Autodesk Inventor part; units mm, degrees
ref_plane "Work Plane1" through (-16.584, 2, -16.584) normal (0, 1, 0) x (0.3814, 0, 0.9244)
ref_plane "YZ Plane" through (0, 0, 0) normal (1, 0, 0) x (0, 1, 0)
ref_plane "XZ Plane" through (0, 0, 0) normal (0, 1, 0) x (-1, 0, 0)
ref_plane "Work Plane1" through (-16.584, 2, -16.584) normal (0, 1, 0) x (0.3814, 0, 0.9244)
sketch "Sketch1" plane through (0, 0, 0) normal (0, 1, 0) x (-1, 0, 0)
  circle A0 centre (0, 0) radius 22.5
  circle A1 centre (0, 0) radius 19.5
  circle A2 centre (0, 0) radius 12.7
  circle A3 centre (0, 0) radius 6
  circle A4 centre (8.8049, 3.6331) radius 1.63
  circle A5 centre (7.5488, -5.8087) radius 1.63
  circle A6 centre (-1.2561, -9.4418) radius 1.63
  circle A7 centre (-8.8049, -3.6331) radius 1.63
  circle A8 centre (-7.5488, 5.8087) radius 1.63
  circle A9 centre (1.2561, 9.4418) radius 1.63
  circle A10 centre (0, 0) radius 12.85
  dimension "d0" = 45
  dimension "d1" = 3
  dimension "d4" = 0.15
extrude "Extrusion1" add sketch "Sketch1" along normal blind 2 contours A1
sketch "Sketch4" plane through (0, 2, 0) normal (0, 1, 0) x (1, 0, 0)
  circle A0 centre (0, 0) radius 22.5
  circle A1 centre (0, 0) radius 19.5
  circle A2 centre (0, 0) radius 18.5
  dimension "d13" = 45
  dimension "d14" = 3
  dimension "d15" = 1
extrude "Extrusion4" add sketch "Sketch4" along normal blind 51 contours A1
fillet "Fillet2" radius 1 1 edges at (12.85, 0, 0)
fillet "Fillet3" radius 2 1 edges at (-18.5, 2, 0)
properties part number "tulejka"
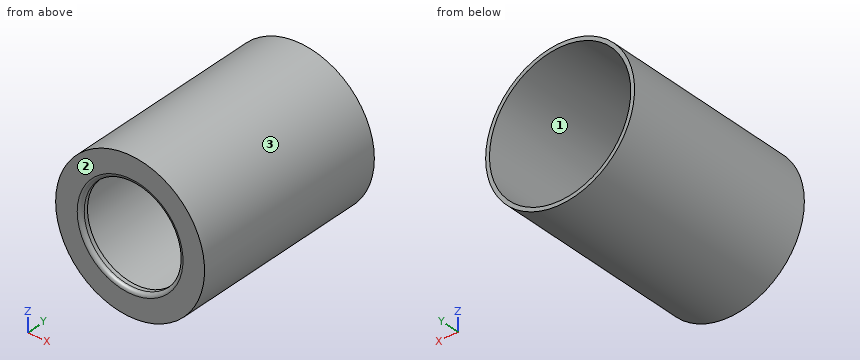
CAD build for the part. Positions are in the model's coordinates, mm. Face numbers are marked on the shaded views. Give positions to 0.01 mm unless a question says otherwise; leave off trailing zeros. Write each loop counter-clockwise with the first axis right and the second up, starting at its lowest first coordinate (ties: lowest second). Pieces come first, ordered by that corner, then holes. Notation, with made-up numbers: (81, -40) - (88, -40) arc R20 cw to (88, -19) - close; hole circle Ø6 at (35.5, -19). An arc over 180 degrees is marked (long way). Put each result on its own line as item: value.
(1) Wall check: L1, parallel to Z at x = 0, y = 1.5; L2, parallel to X at y = 33, z = 0. Give the ranges that are in metal, low to high.
Working result:
L1: -19.5 to -12.85, 12.85 to 19.5
L2: -19.5 to -18.5, 18.5 to 19.5
(2) Saw through at B-B (y = 21.5). List the corners of the cut face in (x, z).
Working result:
outline: circle Ø39 at (0, 0); hole circle Ø37 at (0, 0)
(3) Drop flat-ended pins along their axis: pin 1 Ø3 at (y, z) = (23.5, 14) entering from +X; pin 2 Ø5 at (x, y) = (2, 8.5) entering from -Z; pin 3 Ø1.5 at (x, z) = (13, -13.5) entering from -Y; pin 4 Ø5 at (y, z) = (39, -3.5) entering from -X. Give the stop position or say it passes through.
Working result:
pin 1: x = 14.97
pin 2: z = -19.5
pin 3: y = 0
pin 4: x = -19.47
(4) Pull direction Z, two halves, no side cores. Call the marked faces 1, 2 and 3: released by +Z, released by -Z, zero draft, split by the parting line, or undercut.
Working result:
face 1: undercut
face 2: zero draft
face 3: split by the parting line
